```python
from build123d import *

# Parameters (mm, degrees)
SKETCH_1_R               = 100
EXTRUDE_1_DEPTH          = 5
SKETCH_2_R               = 1.4
CUT_EXTRUDE_1_DEPTH      = 5
SKETCH_4_W               = 5
SKETCH_4_H               = 25
CUT_EXTRUDE_2_DEPTH      = 5
PATTERN_CIRCULAR_2_COUNT = 4
PATTERN_CIRCULAR_2_ANGLE = 135
SKETCH_5_W               = 30
SKETCH_5_H               = 30
SKETCH_5_H_2             = 15
SKETCH_5_W_2             = 15
CUT_EXTRUDE_3_DEPTH      = 5


with BuildPart() as part:
    # 草图1 → 凸台-拉伸1 (new body)
    with BuildSketch(Plane(origin=(0, 0, 0), x_dir=(1, 0, 0), z_dir=(0, 1, 0))):
        Circle(SKETCH_1_R)
    extrude(amount=EXTRUDE_1_DEPTH)

    # 草图2 → 切除-拉伸1 (cut)
    with BuildSketch(Plane(origin=(0, 5, 0), x_dir=(1, 0, 0), z_dir=(0, 1, 0))):
        with Locations((28, 28)):
            Circle(SKETCH_2_R)
        with Locations((28, -28)):
            Circle(SKETCH_2_R)
        with Locations((-28, -28)):
            Circle(SKETCH_2_R)
        with Locations((-28, 28)):
            Circle(SKETCH_2_R)
    extrude(amount=-CUT_EXTRUDE_1_DEPTH, mode=Mode.SUBTRACT)

    # 草图4 → 切除-拉伸2 (cut)
    with BuildSketch(Plane(origin=(0, 5, 0), x_dir=(1, 0, 0), z_dir=(0, 1, 0))):
        with Locations((0, 72.2)):
            Rectangle(SKETCH_4_W, SKETCH_4_H)
        with Locations((0, -72.2)):
            Rectangle(SKETCH_4_W, SKETCH_4_H)
    cut_extrude_2 = extrude(amount=-CUT_EXTRUDE_2_DEPTH, mode=Mode.SUBTRACT)

    # 阵列(圆周)2: 切除-拉伸2 ×4 about axis
    pattern_circular_2_axis = Axis((0, 0, 0), (0, 1, 0))
    for i in range(1, PATTERN_CIRCULAR_2_COUNT):
        add(cut_extrude_2.rotate(pattern_circular_2_axis, i * PATTERN_CIRCULAR_2_ANGLE / (PATTERN_CIRCULAR_2_COUNT - 1)), mode=Mode.SUBTRACT)

    # 草图5 → 切除-拉伸3 (cut)
    with BuildSketch(Plane(origin=(0, 5, 0), x_dir=(1, 0, 0), z_dir=(0, 1, 0))):
        Rectangle(SKETCH_5_W, SKETCH_5_H)
        with Locations((0, 22.5)):
            Rectangle(SKETCH_5_W, SKETCH_5_H_2)
        with Locations((22.5, 0)):
            Rectangle(SKETCH_5_W_2, SKETCH_5_H)
        with Locations((0, -22.5)):
            Rectangle(SKETCH_5_W, SKETCH_5_H_2)
        with Locations((-22.5, 0)):
            Rectangle(SKETCH_5_W_2, SKETCH_5_H)
    extrude(amount=-CUT_EXTRUDE_3_DEPTH, mode=Mode.SUBTRACT)


solid = part.part
```
Geometry: final body of the model. Coordinates: model frame, mm. Coordinates: 2 decimals unless noted, no trailing zeros. Order: outer loops, then holes, each group sorted by start corner. A loop starts at its lowest first (then second) coordinate and runs counter-clockwise, first axis right, second up. Notation, with made-up numbers: (85.25, -27) -> (108.25, -27) arc R14 ccw to (108.25, -1) -> close; hole circle Ø6 at (55, -26.75). An arc over 180 degrees is marked (long way). Write each question's results on one line, items separated by ' | '. Start each with the question number.
1) Material intervals for line 1 along Z through (x, y) = (-52.5, 3.6); line 2 along X through (y, z) = (3.8, 0); line 3 along X through (y, z) = (1.4, -28), sorted ascending.
2) Cut plane C-C, the plane y = 1.65. State how many separate pieces and enclosed holes the cut face has, and give its area (3 significant figures).
3) First-contact query: pin 1 (2 mm diameter, centred on x = 29.5, y = 4, fed in from -Z); pin 2 (1.5 mm diameter, centred on x = -22, y = 3, fed in from +Z); pin 3 (2.5 mm diameter, centred on y = 2, z = 68, fed in from -X). Flat tips, straight axial feed; report the tip coordinate or a pass-through.
4) Cut plane D-D, the plane z = -20. Output: boundary loops of the cut face in (x, y).
5) Cut plane A-A, the plane z = 0. Output: boundary loops of the cut face in (x, y), and give its area (3 significant figures).
6) Cut plane B-B, the plane x = 0. Output: boundary loops of the cut face in (y, z), and give its area (3 significant figures).
7) Mould query, pull axis X, two halves, no side actions, for faces 1 (the flat face through (21, 0, 21)), 2 (the flat face through (-72, 3, 2.5)), 3 (the flat face through (0, 3, -30)). Classes: released by +X, released by -X, zero draft, split by the parting line, or undercut.
Checks:
1) line 1: -85.11 to -56.04, -48.96 to 48.96, 56.04 to 85.11 | line 2: -100 to -84.7, -59.7 to -30, 30 to 59.7, 84.7 to 100 | line 3: -96 to -29.4, -26.6 to -15, 15 to 26.6, 29.4 to 96
2) separate pieces: 1 | enclosed holes: 13 | area: 27,700 mm^2
3) pin 1: z = -95.85 | pin 2: z = 97.72 | pin 3: x = -74.46
4) outline: (-97.98, 0) -> (-15, 0) -> (-15, 5) -> (-97.98, 5) -> close; (15, 0) -> (97.98, 0) -> (97.98, 5) -> (15, 5) -> close
5) outline: (-100, 0) -> (-84.7, 0) -> (-84.7, 5) -> (-100, 5) -> close; (-59.7, 0) -> (-30, 0) -> (-30, 5) -> (-59.7, 5) -> close; (30, 0) -> (59.7, 0) -> (59.7, 5) -> (30, 5) -> close; (84.7, 0) -> (100, 0) -> (100, 5) -> (84.7, 5) -> close | area: 450 mm^2
6) outline: (0, -100) -> (5, -100) -> (5, -84.7) -> (0, -84.7) -> close; (0, -59.7) -> (5, -59.7) -> (5, -30) -> (0, -30) -> close; (0, 30) -> (5, 30) -> (5, 59.7) -> (0, 59.7) -> close; (0, 84.7) -> (5, 84.7) -> (5, 100) -> (0, 100) -> close | area: 450 mm^2
7) face 1: zero draft | face 2: undercut | face 3: undercut
